```python
from build123d import *

# Parameters (mm, degrees)
SKETCH1_R           = 2.0955
BOSS_EXTRUDE1_DEPTH = 2.794
SKETCH2_R           = 42.545
CUT_EXTRUDE2_DEPTH  = 3.794
SKETCH4_W           = 31.35
SKETCH4_H           = 81.35
BOSS_EXTRUDE3_DEPTH = 3.81
CIRPATTERN1_COUNT   = 2
SKETCH5_W           = 25.5
SKETCH5_H           = 75.5
CUT_EXTRUDE3_DEPTH  = 0.5
CUT_EXTRUDE5_REACH  = 5.81
SKETCH24_W          = 31.35
SKETCH24_H          = 59.718160102
CUT_EXTRUDE6_START  = -3.31
SKETCH25_R          = 31.999566145
CUT_EXTRUDE6_DEPTH  = 3.31


with BuildPart() as part:
    # Sketch1 → Boss-Extrude1 (new body)
    with BuildSketch(Plane(origin=(0, 0, 0), x_dir=(1, 0, 0), z_dir=(0, 1, 0))):
        with BuildLine():
            Line((46.558969061, 6.35), (52.908969061, 6.35))
            ThreePointArc((52.908969061, 6.35), (59.258969061, 0), (52.908969061, -6.35))
            Line((52.908969061, -6.35), (46.558969061, -6.35))
            ThreePointArc((46.558969061, -6.35), (33.226947648, -33.226947648), (6.35, -46.558969061))
            Line((6.35, -46.558969061), (6.35, -52.908969061))
            ThreePointArc((6.35, -52.908969061), (0, -59.258969061), (-6.35, -52.908969061))
            Line((-6.35, -52.908969061), (-6.35, -46.558969061))
            ThreePointArc((-6.35, -46.558969061), (-33.226947648, -33.226947648), (-46.558969061, -6.35))
            Line((-46.558969061, -6.35), (-52.908969061, -6.35))
            ThreePointArc((-52.908969061, -6.35), (-59.258969061, 0), (-52.908969061, 6.35))
            Line((-52.908969061, 6.35), (-46.558969061, 6.35))
            ThreePointArc((-46.558969061, 6.35), (-33.226947648, 33.226947648), (-6.35, 46.558969061))
            Line((-6.35, 46.558969061), (-6.35, 52.908969061))
            ThreePointArc((-6.35, 52.908969061), (0, 59.258969061), (6.35, 52.908969061))
            Line((6.35, 52.908969061), (6.35, 46.558969061))
            ThreePointArc((6.35, 46.558969061), (33.226947648, 33.226947648), (46.558969061, 6.35))
        make_face()
        with Locations((52.908969061, 0)):
            Circle(SKETCH1_R, mode=Mode.SUBTRACT)
        with Locations((0, -52.908969061)):
            Circle(SKETCH1_R, mode=Mode.SUBTRACT)
        with Locations((-52.908969061, 0)):
            Circle(SKETCH1_R, mode=Mode.SUBTRACT)
        with Locations((0, 52.908969061)):
            Circle(SKETCH1_R, mode=Mode.SUBTRACT)
    extrude(amount=BOSS_EXTRUDE1_DEPTH)

    # Sketch2 → Cut-Extrude2 (cut, through all)
    with BuildSketch(Plane(origin=(0, 2.794, 0), x_dir=(1, 0, 0), z_dir=(0, 1, 0))):
        Circle(SKETCH2_R)
    extrude(amount=-CUT_EXTRUDE2_DEPTH, mode=Mode.SUBTRACT)



with BuildPart() as body_2:
    # Sketch4 → Boss-Extrude3 (new body)
    with BuildSketch(Plane(origin=(0, 21.336, 0), x_dir=(-1, 0, 0), z_dir=(0, -1, 0))):
        Rectangle(SKETCH4_W, SKETCH4_H)
    extrude(amount=BOSS_EXTRUDE3_DEPTH)


with BuildPart() as part_1:
    add(part.part)

    add(body_2.part)  # Sweep2 merges body 2
    # Sweep2: sweep along a path in Sketch22
    with BuildLine(Plane(origin=(0, 2.794, 0), x_dir=(1, 0, 0), z_dir=(0, 1, 0))) as sweep2_path:
        ThreePointArc((15.298922649, 39.699118262), (0, 42.545), (-15.298922649, 39.699118262))
    # Sketch6 → Sweep2 (sweep)
    with BuildSketch(Plane(origin=(0, 0, 0), x_dir=(0.359593904, 0, -0.933108903), z_dir=(0.933108903, 0, 0.359593904))):
        with BuildLine():
            Line((46.99, 2.794), (42.545, 2.794))
            add(Edge.make_bspline(
                [(42.545, 2.794), (38.735, 5.334), (29.845, 21.336)],
                knots=[0, 0, 0, 1, 1, 1], degree=2))
            Line((29.845, 21.336), (43.590839061, 21.336))
            add(Edge.make_bspline(
                [(43.590839061, 21.336), (43.590839061, 5.334), (46.99, 2.794)],
                knots=[0, 0, 0, 1, 1, 1], degree=2))
        make_face()
    sweep2 = sweep(path=sweep2_path.line)

    # CirPattern1: Sweep2 ×2 about axis
    cirpattern1_axis = Axis((0, 0, 0), (0, -1, 0))
    for i in range(1, CIRPATTERN1_COUNT):
        add(sweep2.rotate(cirpattern1_axis, i * 360 / CIRPATTERN1_COUNT))

    # Sketch5 → Cut-Extrude3 (cut)
    with BuildSketch(Plane(origin=(0, 21.336, 0), x_dir=(1, 0, 0), z_dir=(0, 1, 0))):
        Rectangle(SKETCH5_W, SKETCH5_H)
    extrude(amount=-CUT_EXTRUDE3_DEPTH, mode=Mode.SUBTRACT)

    # Sketch24 → Cut-Extrude5 (cut, up to next)
    with BuildSketch(Plane.XZ.offset(-17.526), mode=Mode.PRIVATE) as cut_extrude5_sk1:
        Rectangle(SKETCH24_W, SKETCH24_H)
    cut_extrude5_tool1 = extrude(cut_extrude5_sk1.sketch, amount=-CUT_EXTRUDE5_REACH, mode=Mode.PRIVATE) & part_1.part
    add(cut_extrude5_tool1.solids().sort_by_distance((0, 17.526, 0))[0], mode=Mode.SUBTRACT)

    # Sketch25 → Cut-Extrude6 (cut)
    with BuildSketch(Plane.XZ.offset(-17.526).offset(CUT_EXTRUDE6_START)):
        Circle(SKETCH25_R)
    extrude(amount=CUT_EXTRUDE6_DEPTH, mode=Mode.SUBTRACT)


solid = part_1.part
```
Can you work these out from the model? Positions are in its coordinate system, mm. A direction names the side the tool comes from. Give positions to 0.01 mm unless a question says otherwise; leave off trailing zeros. Loops run counter-clockwise (first coordinate to the right, second up) from the corner with the lowest first, then second, coordinate; pieces in that order, holes last. Notation, with made-up numbers: M 34,38.5 L 53,38.5 A17 cw 53,54.5 Z; hole C 84,0 d1. An arc over 180 degrees is marked long. One line per question, with ' | ' between items. Start each with the question number.
Q1. For faces 1 (the flat face through (-6.35, 1, -50)), 2 (the flat face through (-14, 19, 29.859)), 3 (the flat face through (-6.35, 1, 50)), 4 (the flat face through (-14.24, 11.94, 36.95)), which set-ups out of +Z, -Z, +X, -X, +Y, -Y let a thin tool reach every point of the face, with its end or its side?
Q2. If I drill on line 1 (Z direction, x = 0, y = 1.35) (3 decimals); line 2 (Y direction, x = 43, z = -18.5), over which ranges is the centre line in solid material (lowest first)? Write a range as from..to.
Q3. If we section it at C-C (z = 15): Please give me the cut outline in (x, y).
Q4. If we section it at D-D (x = 0): State how many separate pieces and enclosed holes the cut face has, plus the area to 3 significant figures.
Q5. For pin 1 Ø1.4 at (y, z) = (1.5, -49) entering from +X; pin 2 Ø3.5 at (x, z) = (0, -52.91) entering from +Y; pin 3 Ø8 at (x, y) = (-20, 2.5) entering from +Z; pin 4 Ø3.5 at (x, z) = (-14.5, -37) entering from -Y, each with a flat end and sliding along its axis, tell me the tip position at first contact or that it passes through.
Q6. If we section it at A-A (z = 0): Please give me the cut outline in (x, y) (3 decimals), plus the area to 3 significant figures.
Q7. If we mould it in two halves opening along X, with no side actions, what happens to faces 5 (the cylindrical face through (32.92, 1.38, -33.53)), 6 (the cylindrical face through (-33.76, 1.42, 25.89)), 7 (the flat face through (-14.24, 11.94, -36.95))? For each: +X half, -X half, draft (parallel to the pull), parting line (faces both ways), or undercut.
Q8. If we section it at B-B (x = -36): Please give me the cut outline in (y, z), plus the area to 3 significant figures.
Computed:
1) face 1: -Z, -X, +Y, -Y | face 2: +X, -X, +Y, -Y | face 3: +Z, -X, +Y, -Y | face 4: -X
2) line 1: z = -59.259..-55.004, -50.813..-42.545, 42.545..50.813, 55.004..59.259 | line 2: y = 0..2.79
3) outline: M -44.53,0 L -39.81,0 L -39.81,2.79 L -44.53,2.79 Z; M 39.81,0 L 44.53,0 L 44.53,2.79 L 39.81,2.79 Z
4) separate pieces: 4 | enclosed holes: 0 | area: 383 mm²
5) pin 1: stops at x = 6.35 | pin 2: passes through | pin 3: stops at z = 44.18 | pin 4: stops at y = 3.68
6) outline: M -59.259,0 L -55.004,0 L -55.004,2.794 L -59.259,2.794 Z; M -50.813,0 L -42.545,0 L -42.545,2.794 L -50.813,2.794 Z; M 42.545,0 L 50.813,0 L 50.813,2.794 L 42.545,2.794 Z; M 55.004,0 L 59.259,0 L 59.259,2.794 L 55.004,2.794 Z | area: 70.0 mm²
7) face 5: +X half | face 6: undercut | face 7: -X half
8) outline: M 0,-30.2 L 2.79,-30.2 L 2.79,-22.67 L 0,-22.67 Z; M 0,22.67 L 2.79,22.67 L 2.79,30.2 L 0,30.2 Z | area: 42.1 mm²
